```python
from build123d import *

# Parameters (mm, degrees)
BOSS_EXTRUDE1_DEPTH = 45
BOSS_EXTRUDE2_DEPTH = 5
CUT_EXTRUDE1_REACH  = 148.924
SKETCH3_R           = 10.5
SKETCH5_W           = 20
SKETCH5_H           = 30
BOSS_EXTRUDE3_DEPTH = 10
SKETCH6_R           = 5.087291531
CUT_EXTRUDE2_DEPTH  = 10
SKETCH8_W           = 10
SKETCH8_H           = 56
BOSS_EXTRUDE4_DEPTH = 90
FILLET1_R           = 10
FILLET2_R           = 10
FILLET3_R           = 2
SKETCH9_W           = 10
SKETCH9_H           = 15
BOSS_EXTRUDE5_DEPTH = 30
FILLET4_R           = 10
FILLET5_R           = 5


with BuildPart() as part:
    # Sketch1 → Boss-Extrude1 (new, symmetric)
    with BuildSketch(Plane.XY):
        Polygon((41.677960524, 0), (-38.322039476, 60), (-48.322039476, 60), (-48.322039476, 64), (-36.988706143, 64), (43.011293857, 4), (51.677960524, 4), (51.677960524, 0), align=None)
    extrude(amount=BOSS_EXTRUDE1_DEPTH, both=True)

    # Sketch2 → Boss-Extrude2 (add)
    with BuildSketch(Plane.XY.offset(45)):
        Polygon((-48.322039476, 64), (-48.322039476, 104), (-36.988706143, 104), (43.011293857, 44), (51.677960524, 44), (51.677960524, 4), (43.011293857, 4), (-36.988706143, 64), align=None)
    boss_extrude2 = extrude(amount=-BOSS_EXTRUDE2_DEPTH)

    # Mirror1: Boss-Extrude2 across plane
    add(boss_extrude2.mirror(Plane.XY))

    # Sketch3 → Cut-Extrude1 (cut, up to next)
    with BuildSketch(Plane(origin=(0, 0, -45), x_dir=(-1, 0, 0), z_dir=(0, 0, -1)), mode=Mode.PRIVATE) as cut_extrude1_sk1:
        with Locations((-21.677960524, 38)):
            Circle(SKETCH3_R)
    cut_extrude1_tool1 = extrude(cut_extrude1_sk1.sketch, amount=-CUT_EXTRUDE1_REACH, mode=Mode.PRIVATE) & part.part
    add(cut_extrude1_tool1.solids().sort_by_distance((21.677961, 38, -45))[0], mode=Mode.SUBTRACT)

    # Sketch5 → Boss-Extrude3 (add)
    with BuildSketch(Plane.ZY.offset(48.322039476)):
        with Locations((0, 45)):
            Rectangle(SKETCH5_W, SKETCH5_H)
    extrude(amount=-BOSS_EXTRUDE3_DEPTH)

    # Sketch6 → Cut-Extrude2 (cut)
    with BuildSketch(Plane.ZY.offset(48.322039476)):
        with Locations((0, 44)):
            Circle(SKETCH6_R)
    extrude(amount=-CUT_EXTRUDE2_DEPTH, mode=Mode.SUBTRACT)

    # Sketch8 → Boss-Extrude4 (add)
    with BuildSketch(Plane.XY.offset(45)):
        with Locations((46.677960524, -28)):
            Rectangle(SKETCH8_W, SKETCH8_H)
    extrude(amount=-BOSS_EXTRUDE4_DEPTH)

    # Fillet1
    fillet1_edges = [part.edges().sort_by_distance(p)[0] for p in [
        (-43.322039476, 60, -10),
        (-43.322039476, 60, 10),
    ]]
    fillet(fillet1_edges, radius=FILLET1_R)

    # Fillet2
    fillet2_edges = [part.edges().sort_by_distance(p)[0] for p in [
        (41.677960524, 0, 0),
    ]]
    fillet(fillet2_edges, radius=FILLET2_R)

    # Fillet3
    fillet3_edges = [part.edges().sort_by_distance(p)[0] for p in [
        (-48.322039476, 84, 40),
        (-48.322039476, 104, 42.5),
        (47.344627191, 44, 45),
        (3.011293857, 74, 45),
        (-42.655372809, 104, 45),
        (47.344627191, 44, -45),
        (3.011293857, 74, -45),
        (-42.655372809, 104, -45),
        (-48.322039476, 104, -42.5),
        (-48.322039476, 84, -40),
    ]]
    fillet(fillet3_edges, radius=FILLET3_R)

    # Sketch9 → Boss-Extrude5 (add)
    with BuildSketch(Plane(origin=(0, 0, -45), x_dir=(-1, 0, 0), z_dir=(0, 0, -1))):
        with Locations((-46.677960524, -48.5)):
            Rectangle(SKETCH9_W, SKETCH9_H)
    extrude(amount=BOSS_EXTRUDE5_DEPTH)

    # Fillet4
    fillet4_edges = [part.edges().sort_by_distance(p)[0] for p in [
        (46.677960524, -41, -45),
    ]]
    fillet(fillet4_edges, radius=FILLET4_R)

    # Fillet5
    fillet5_edges = [part.edges().sort_by_distance(p)[0] for p in [
        (46.677960524, -41, -75),
    ]]
    fillet(fillet5_edges, radius=FILLET5_R)


solid = part.part
```
Part model, mm, in its own coordinate system. A direction names the side the tool comes from. Round coordinates to 2 decimals unless told otherwise and drop trailing zeros. Write each loop counter-clockwise with the first axis right and the second up, starting at its lowest first coordinate (ties: lowest second). Pieces come first, ordered by that corner, then holes. Notation, with made-up numbers: (74, -18) -> (94, -18) arc R13 ccw to (94, -10) -> close; hole circle Ø8 at (87, 62). An arc over 180 degrees is marked (long way). Return JSON: item names as keys, results as strings. Group by question number.
Q1. Mould opens along Z. For faces 1 (the flat face through (2.45, 74.42, -41.52)), 2 (the flat face through (47, 4, 1)), 3 (the cylindrical face through (-43.25, 56.99, 12.85)), 4 (the cylindrical face through (-43.25, 57.15, -13.01)) say: pulls with the +Z half, pulls with the -Z half, needs draft (parallel to the pull), parting line crosses it, or undercut.
Q2. Which spindle directions (+Z, -Z, +X, -X, +Y, -Y) get a long thin tool onto all of the face, cutting with end or side? Do faces 5 (the flat face through (2.45, 34.42, 0.56)), 6 (the flat face through (41.678, -31, -1)), 7 (the cylindrical face through (11.98, 33.98, -42.54)). Say none if no direction does.
Q3. Saw through at A-A on z = 0. Write the cut outline in (x, y).
Q4. Pin check, flat tips, straight feed: pin 1 (12 mm diameter, centred on x = -6.5, z = -50, fed in from +Y); pin 2 (5 mm diameter, centred on y = -18.5, z = 26.5, fed in from -X); pin 3 (9 mm diameter, centred on y = 44, z = 0, fed in from -X); pin 4 (12 mm diameter, centred on y = 53.5, z = -52, fed in from +X). Stop position of each tip, or through.
Q5. Saw through at B-B on z = 33. Write the cut outline in (x, y), plus the area to 3 significant figures.
Q6. Saw through at C-C on z = -57. Write the cut outline in (x, y).
Q7. Probe L1, parallel to Y at x = -40.5, z = 0; L2, parallel to Z at x = -14.5, y = 50; L3, parallel to X at y = -6, z = -28. List the from-to ranges inside material, lowest first. Write a range as [from, to].
Answer:
{
 "1": {"face 1": "needs draft", "face 2": "undercut", "face 3": "pulls with the +Z half", "face 4": "pulls with the -Z half"},
 "2": {"face 5": "+X, +Y", "face 6": "+Z, -Z, -X, -Y", "face 7": "-Z"},
 "3": {"outline": "(-48.32, 30) -> (-38.32, 30) -> (-38.32, 38.91) -> (-48.32, 38.91) -> close; (-48.32, 49.09) -> (-38.32, 49.09) -> (-38.32, 60) -> (37.68, 3) arc R10 cw to (41.68, -5) -> (41.68, -56) -> (51.68, -56) -> (51.68, 4) -> (43.01, 4) -> (-36.99, 64) -> (-48.32, 64) -> close"},
 "4": {"pin 1": "y = 82.1", "pin 2": "x = 41.68", "pin 3": "x = -22.99", "pin 4": "through"},
 "5": {"outline": "(-48.32, 60) -> (-38.32, 60) -> (37.68, 3) arc R10 cw to (41.68, -5) -> (41.68, -56) -> (51.68, -56) -> (51.68, 4) -> (43.01, 4) -> (-36.99, 64) -> (-48.32, 64) -> close", "area": "1,040 mm2"},
 "6": {"outline": "(41.68, -56) -> (51.68, -56) -> (51.68, -41) -> (41.68, -41) -> close"},
 "7": {"L1": "[30, 38.91], [49.09, 64]", "L2": "[-45, -40], [40, 45]", "L3": "[41.68, 51.68]"}
}
